from build123d import *

# Parameters (mm, degrees)
SKETCH1_W            = 8.5
SKETCH1_H            = 8.5
BOSS_EXTRUDE1_DEPTH  = 5
SKETCH2_W            = 8.5
SKETCH2_H            = 8.5
BOSS_EXTRUDE2_DEPTH  = 2
SKETCH3_R            = 1.5
CUT_EXTRUDE1_DEPTH   = 2
SKETCH4_W            = 81.5
SKETCH4_H            = 8.5
BOSS_EXTRUDE3_DEPTH  = 3
SKETCH5_W            = 7
SKETCH5_H            = 8.5
BOSS_EXTRUDE4_DEPTH  = 8.5
CUT_EXTRUDE2_DEPTH   = 5
SKETCH7_R            = 1.5
CUT_EXTRUDE3_DEPTH   = 5
CUT_EXTRUDE4_DEPTH   = 10
SKETCH9_W            = 8.5
SKETCH9_H            = 8.5
SKETCH9_R            = 1.5
BOSS_EXTRUDE5_DEPTH  = 2
CUT_EXTRUDE5_DEPTH   = 2
SKETCH11_W           = 8.5
SKETCH11_H           = 8.5
SKETCH11_R           = 1.5
BOSS_EXTRUDE6_DEPTH  = 2
BOSS_EXTRUDE7_DEPTH  = 5
BOSS_EXTRUDE8_DEPTH  = 5
SKETCH14_W           = 8.5
SKETCH14_H           = 11.5
CUT_EXTRUDE6_DEPTH   = 4
SKETCH15_W           = 8.5
SKETCH15_H           = 11.5
CUT_EXTRUDE7_DEPTH   = 4
SKETCH16_R           = 1.5
CUT_EXTRUDE8_DEPTH   = 4
SKETCH17_R           = 1.5
CUT_EXTRUDE9_DEPTH   = 4
SKETCH19_W           = 8.5
SKETCH19_H           = 8.5
BOSS_EXTRUDE9_DEPTH  = 3
SKETCH20_W           = 8.5
SKETCH20_H           = 8.5
BOSS_EXTRUDE10_DEPTH = 3


with BuildPart() as part:
    # Sketch1 → Boss-Extrude1 (new body)
    with BuildSketch(Plane(origin=(0, 0, 0), x_dir=(0, 0, -1), z_dir=(1, 0, 0))):
        Rectangle(SKETCH1_W, SKETCH1_H)
        Polygon((1.58771324, 2.75), (-1.58771324, 2.75), (-3.175426481, 0), (-1.58771324, -2.75), (1.58771324, -2.75), (3.175426481, 0), align=None, mode=Mode.SUBTRACT)
    extrude(amount=BOSS_EXTRUDE1_DEPTH)

    # Sketch2 → Boss-Extrude2 (add)
    with BuildSketch(Plane.ZY):
        Rectangle(SKETCH2_W, SKETCH2_H)
    extrude(amount=BOSS_EXTRUDE2_DEPTH)

    # Sketch3 → Cut-Extrude1 (cut)
    with BuildSketch(Plane(origin=(0, 0, 0), x_dir=(0, 0, -1), z_dir=(1, 0, 0))):
        Circle(SKETCH3_R)
    extrude(amount=-CUT_EXTRUDE1_DEPTH, mode=Mode.SUBTRACT)

    # Sketch4 → Boss-Extrude3 (add)
    with BuildSketch(Plane.XZ.offset(4.25)):
        with Locations((38.75, 0)):
            Rectangle(SKETCH4_W, SKETCH4_H)
    extrude(amount=BOSS_EXTRUDE3_DEPTH)

    # Sketch5 → Boss-Extrude4 (add)
    with BuildSketch(Plane(origin=(0, -4.25, 0), x_dir=(1, 0, 0), z_dir=(0, 1, 0))):
        with Locations((76, 0)):
            Rectangle(SKETCH5_W, SKETCH5_H)
    extrude(amount=BOSS_EXTRUDE4_DEPTH)

    # Sketch6 → Cut-Extrude2 (cut)
    with BuildSketch(Plane.ZY.offset(-72.5)):
        Polygon((3.175426481, 0), (1.58771324, 2.75), (-1.58771324, 2.75), (-3.175426481, 0), (-1.58771324, -2.75), (1.58771324, -2.75), align=None)
    extrude(amount=-CUT_EXTRUDE2_DEPTH, mode=Mode.SUBTRACT)

    # Sketch7 → Cut-Extrude3 (cut)
    with BuildSketch(Plane.ZY.offset(-77.5)):
        Circle(SKETCH7_R)
    extrude(amount=-CUT_EXTRUDE3_DEPTH, mode=Mode.SUBTRACT)

    # Sketch8 → Cut-Extrude4 (cut)
    with BuildSketch(Plane.ZY.offset(2)):
        Polygon((-1.58771324, 2.75), (1.58771324, 2.75), (3.175426481, 0), (1.58771324, -2.75), (-1.58771324, -2.75), (-3.175426481, 0), align=None)
    extrude(amount=-CUT_EXTRUDE4_DEPTH, mode=Mode.SUBTRACT)

    # Sketch9 → Boss-Extrude5 (add)
    with BuildSketch(Plane(origin=(5, 0, 0), x_dir=(0, 0, -1), z_dir=(1, 0, 0))):
        Rectangle(SKETCH9_W, SKETCH9_H)
        Circle(SKETCH9_R, mode=Mode.SUBTRACT)
    extrude(amount=-BOSS_EXTRUDE5_DEPTH)

    # Sketch10 → Cut-Extrude5 (cut)
    with BuildSketch(Plane(origin=(79.5, 0, 0), x_dir=(0, 0, -1), z_dir=(1, 0, 0))):
        Polygon((-3.175426481, 0), (-1.58771324, 2.75), (1.58771324, 2.75), (3.175426481, 0), (1.58771324, -2.75), (-1.58771324, -2.75), align=None)
    extrude(amount=-CUT_EXTRUDE5_DEPTH, mode=Mode.SUBTRACT)

    # Sketch11 → Boss-Extrude6 (add)
    with BuildSketch(Plane.ZY.offset(-72.5)):
        Rectangle(SKETCH11_W, SKETCH11_H)
        Circle(SKETCH11_R, mode=Mode.SUBTRACT)
    extrude(amount=-BOSS_EXTRUDE6_DEPTH)

    # Sketch12 → Boss-Extrude7 (add)
    with BuildSketch(Plane.ZY.offset(-3)):
        Polygon((-3.175426481, 0), (-1.58771324, 2.75), (1.58771324, 2.75), (3.175426481, 0), (1.58771324, -2.75), (-1.58771324, -2.75), align=None)
    extrude(amount=BOSS_EXTRUDE7_DEPTH)

    # Sketch13 → Boss-Extrude8 (add)
    with BuildSketch(Plane(origin=(74.5, 0, 0), x_dir=(0, 0, -1), z_dir=(1, 0, 0))):
        Polygon((-1.58771324, 2.75), (-3.175426481, 0), (-1.58771324, -2.75), (1.58771324, -2.75), (3.175426481, 0), (1.58771324, 2.75), align=None)
    extrude(amount=BOSS_EXTRUDE8_DEPTH)

    # Sketch14 → Cut-Extrude6 (cut)
    with BuildSketch(Plane.ZY.offset(2)):
        with Locations((0, -1.5)):
            Rectangle(SKETCH14_W, SKETCH14_H)
    extrude(amount=-CUT_EXTRUDE6_DEPTH, mode=Mode.SUBTRACT)

    # Sketch15 → Cut-Extrude7 (cut)
    with BuildSketch(Plane(origin=(79.5, 0, 0), x_dir=(0, 0, -1), z_dir=(1, 0, 0))):
        with Locations((0, -1.5)):
            Rectangle(SKETCH15_W, SKETCH15_H)
    extrude(amount=-CUT_EXTRUDE7_DEPTH, mode=Mode.SUBTRACT)

    # Sketch16 → Cut-Extrude8 (cut)
    with BuildSketch(Plane(origin=(5, 0, 0), x_dir=(0, 0, -1), z_dir=(1, 0, 0))):
        Circle(SKETCH16_R)
    extrude(amount=-CUT_EXTRUDE8_DEPTH, mode=Mode.SUBTRACT)

    # Sketch17 → Cut-Extrude9 (cut)
    with BuildSketch(Plane.ZY.offset(-74.5)):
        Circle(SKETCH17_R)
    extrude(amount=-CUT_EXTRUDE9_DEPTH, mode=Mode.SUBTRACT)

    # Sketch19 → Boss-Extrude9 (add)
    with BuildSketch(Plane(origin=(5, 0, 0), x_dir=(0, 0, -1), z_dir=(1, 0, 0))):
        Rectangle(SKETCH19_W, SKETCH19_H)
    extrude(amount=-BOSS_EXTRUDE9_DEPTH)

    # Sketch20 → Boss-Extrude10 (add)
    with BuildSketch(Plane.ZY.offset(-72.5)):
        Rectangle(SKETCH20_W, SKETCH20_H)
    extrude(amount=-BOSS_EXTRUDE10_DEPTH)


solid = part.part
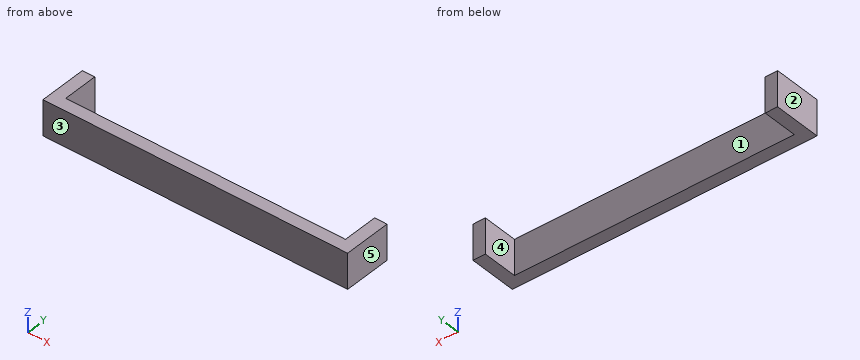
Verification items for the finished model (mm, model axes). Face numbers are marked on the shaded views. A direction names the side the tool comes from. Give positions to 0.01 mm unless a question says otherwise; leave off trailing zeros. Order: outer loops, then holes, each group sorted by start corner. A loop starts at its lowest first (then second) coordinate and runs counter-clockwise, first axis right, second up. Notation, with made-up numbers: M 53,-28.75 L 90,-28.75 A27 cw 90,9.25 Z; hole C 47.25,13 d7. An arc over 180 degrees is marked long. Use one line per item in the form item = value. Start each with the question number.
Q1. Access from +Z, -Z, +X, -X, +Y, -Y to the whole of each face (thin tool, end or side, straight path). Record for the marked faces 1 and 2.
Q2. Mould release check, pull along X, two halves, no side actions. Record for the marked faces 3, 4 and 5: +X half, -X half, draft (parallel to the pull), parting line (faces both ways), or undercut.
Q3. Scan lines: line 1 along X through (y, z) = (-1.75, 2); line 2 along Y through (x, z) = (10.5, 2.5). Record each from-to range of solid material in increasing order. Write a range as [from, to].
Q4. Section check B-B (z = -1). Enter the section's corners in (x, y), then the cut area to 4 significant figures.
Q5. Section check C-C (x = 51). Enter the section's corners in (y, z), then the cut area to 3 significant figures.
Q6. Section check A-A (y = 1). Enter the section's corners in (x, z), then the cut area to 3 significant figures.
Evaluation:
q1.face_1 = +Z, -Z, +Y
q1.face_2 = +Z, -Z, -X, +Y, -Y
q2.face_3 = draft
q2.face_4 = undercut
q2.face_5 = +X half
q3.line_1 = [2, 5], [72.5, 75.5]
q3.line_2 = [-7.25, -4.25]
q4.outline = M 2,-7.25 L 75.5,-7.25 L 75.5,4.25 L 72.5,4.25 L 72.5,-4.25 L 5,-4.25 L 5,4.25 L 2,4.25 Z
q4.area = 271.5 mm2
q5.outline = M -7.25,-4.25 L -4.25,-4.25 L -4.25,4.25 L -7.25,4.25 Z
q5.area = 25.5 mm2
q6.outline = M 2,-4.25 L 5,-4.25 L 5,4.25 L 2,4.25 Z; M 72.5,-4.25 L 75.5,-4.25 L 75.5,4.25 L 72.5,4.25 Z
q6.area = 51.0 mm2
